from build123d import *

# Parameters (mm, degrees)
BOSS_EXTRUDE1_DEPTH = 6.35
SKETCH2_R           = 0.635
CUT_EXTRUDE1_DEPTH  = 7.35
FILLET2_R           = 1.016
FILLET3_R           = 25.4


with BuildPart() as part:
    # Sketch1 → Boss-Extrude1 (new body)
    with BuildSketch(Plane.XY):
        with BuildLine():
            ThreePointArc((-38.731808071, 42.023440406), (-54.328419489, -17.735426012), (-6.477, -56.781783796))
            Line((-6.477, -56.781783796), (6.477, -56.781783796))
            Line((6.477, -56.781783796), (16.637, -56.781783796))
            Line((16.637, -56.781783796), (16.637, -50.431783796))
            Line((16.637, -50.431783796), (6.477, -50.431783796))
            Line((6.477, -50.431783796), (6.477, -53.682983796))
            Line((6.477, -53.682983796), (-6.477, -53.682983796))
            Line((-6.477, -53.682983796), (-6.477, -50.385399383))
            ThreePointArc((-6.477, -50.385399383), (-48.394630123, -15.446675216), (-34.469665313, 37.315977453))
            ThreePointArc((-34.469665313, 37.315977453), (-33.658259426, 39.020726685), (-34.247395693, 40.814456854))
            Line((-34.247395693, 40.814456854), (-35.064641493, 41.788412472))
            ThreePointArc((-35.064641493, 41.788412472), (-36.847939613, 42.690531433), (-38.731808071, 42.023440406))
        make_face()
    extrude(amount=BOSS_EXTRUDE1_DEPTH)

    # Sketch2 → Cut-Extrude1 (cut, through all)
    with BuildSketch(Plane.XY.offset(6.35)):
        with Locations((-6.477, -53.047983796)):
            Circle(SKETCH2_R)
        with Locations((6.477, -53.047983796)):
            Circle(SKETCH2_R)
    extrude(amount=-CUT_EXTRUDE1_DEPTH, mode=Mode.SUBTRACT)

    # Fillet2
    fillet2_edges = [part.edges().sort_by_distance(p)[0] for p in [
        (-6.477, -52.412983796, 3.175),
        (6.477, -52.412983796, 3.175),
    ]]
    fillet(fillet2_edges, radius=FILLET2_R)

    # Fillet3
    fillet3_edges = [part.edges().sort_by_distance(p)[0] for p in [
        (-6.477, -56.781783796, 3.175),
    ]]
    fillet(fillet3_edges, radius=FILLET3_R)


solid = part.part
Design review of the part built by this model. Coordinates are the model's own, in mm. A direction names the side the tool comes from. Coordinates: 2 decimals unless noted, no trailing zeros. Loops run counter-clockwise (first coordinate to the right, second up) from the corner with the lowest first, then second, coordinate; pieces in that order, holes last.
Item 1: For faces 1 (the flat face through (6, -56.782, 3)), 2 (the flat face through (12, -50.432, 3)), list the 3-axis set-ups (+Z, -Z, +X, -X, +Y, -Y) from which the entire face can be reached by the end or side of a thin tool; tool diameter is ignored.
Completed:
face 1: +Z, -Z, +X, -X, -Y
face 2: +Z, -Z, +X, +Y
Item 2: Add section A-A (z = 1.75). Write out the cut boundary in (x, y) (3 decimals), and give its area (3 significant figures).
Completed:
outline: (-38.732, 42.023) arc R57.15 ccw to (-8.679, -56.487) arc R25.4 ccw to (-4.821, -56.782) - (16.637, -56.782) - (16.637, -50.432) - (6.477, -50.432) - (6.477, -51.747) arc R1.016 ccw to (6.868, -52.547) arc R0.635 cw to (6.477, -53.683) - (-6.477, -53.683) arc R0.635 cw to (-6.868, -52.547) arc R1.016 ccw to (-6.477, -51.747) - (-6.477, -50.385) arc R50.8 cw to (-34.47, 37.316) arc R2.54 ccw to (-34.247, 40.814) - (-35.065, 41.788) arc R2.54 ccw to start
area: 897 mm2
Item 3: Clearance check with flat-ended pins moving along their axes: pin 1 (3 mm diameter, centred on x = 12, z = 3.5, fed in from +Y); pin 2 (2 mm diameter, centred on x = -49, z = 5.5, fed in from +Y); pin 3 (1.5 mm diameter, centred on y = -12.5, z = 1.5, fed in from -X). State where each tip first meets the part, or that it passes through.
Completed:
pin 1: stops at y = -50.43
pin 2: stops at y = 31.02
pin 3: stops at x = -55.93
Item 4: Draft analysis for pull direction X (two halves, no side actions). For faces 3 (the flat face through (16.637, -54, 3)), 4 (the flat face through (0, -53.683, 3)), 5 (the flat face through (-48, -18, 0)), 6 (the cylindrical face through (-36.82, 42.69, 3.13)), state which applies: pulls with the +X half, pulls with the -X half, needs draft (parallel to the pull), parting line crosses it, or undercut.
Completed:
face 3: pulls with the +X half
face 4: undercut
face 5: needs draft
face 6: parting line crosses it
Item 5: Add section B-B (x = -49.5). Write out the cut boundary in (y, z).
Completed:
outline: (-28.56, 0) - (-11.42, 0) - (-11.42, 6.35) - (-28.56, 6.35) - close; (11.42, 0) - (28.56, 0) - (28.56, 6.35) - (11.42, 6.35) - close
Item 6: Add section D-D (x = 11). Write out the cut boundary in (y, z).
Completed:
outline: (-56.78, 0) - (-50.43, 0) - (-50.43, 6.35) - (-56.78, 6.35) - close
Item 7: Add section C-C (y = -27). Write out the cut boundary in (x, z).
Completed:
outline: (-50.37, 0) - (-43.03, 0) - (-43.03, 6.35) - (-50.37, 6.35) - close
Item 8: Wall thickness on L1, parallel to Y at x = 7.5, z = 6; L2, parallel to Y at x = 3, z = 4.75; L3, parallel to X at y = -44, z = 4: over which ranges is each line inside the solid? List them lowest first.
Completed:
L1: y = -56.78 to -50.43
L2: y = -56.78 to -53.68
L3: x = -36.47 to -25.39
